```python
from build123d import *

# Parameters (mm, degrees)
F1_DEPTH = 6.35
F3_DEPTH = 3.175
F4_R     = 3.175
F5_DEPTH = 3.175


with BuildPart() as f1:
    # F0 (on Front) → F1 (new body, symmetric)
    with BuildSketch(Plane.XZ):
        with BuildLine():
            Line((0, 10.922), (0, 0))
            Line((0, 0), (10.922, 0))
            ThreePointArc((10.922, 0), (7.7230202641, 7.7230202641), (0, 10.922))
        make_face()
        with BuildLine():
            Line((10.922, 0), (0, 0))
            Line((0, 0), (0, -6.223))
            Line((0, -6.223), (8.9757648699, -6.223))
            ThreePointArc((8.9757648699, -6.223), (10.4240919966, -3.2601211704), (10.922, 0))
        make_face()
        with BuildLine():
            ThreePointArc((0, 10.922), (-7.7230202641, 7.7230202641), (-10.922, 0))
            Line((-10.922, 0), (0, 0))
            Line((0, 0), (0, 10.922))
        make_face()
        with BuildLine():
            Line((0, 0), (-10.922, 0))
            ThreePointArc((-10.922, 0), (-10.4240919966, -3.2601211704), (-8.9757648699, -6.223))
            Line((-8.9757648699, -6.223), (0, -6.223))
            Line((0, -6.223), (0, 0))
        make_face()
    extrude(amount=F1_DEPTH, both=True)

    # F2 (on face) → F3 (join)
    with BuildSketch(Plane.XZ.offset(6.35)):
        with BuildLine():
            Line((3.175, 0), (0, 0))
            Line((0, 0), (0, -3.175))
            ThreePointArc((0, -3.175), (2.2450640303, -2.2450640303), (3.175, 0))
        make_face()
        with BuildLine():
            Line((0, 3.175), (0, 0))
            Line((0, 0), (3.175, 0))
            ThreePointArc((3.175, 0), (2.2450640303, 2.2450640303), (0, 3.175))
        make_face()
        with BuildLine():
            ThreePointArc((0, 3.175), (-2.2450640303, 2.2450640303), (-3.175, 0))
            Line((-3.175, 0), (0, 0))
            Line((0, 0), (0, 3.175))
        make_face()
        with BuildLine():
            Line((0, 0), (-3.175, 0))
            ThreePointArc((-3.175, 0), (-2.2450640303, -2.2450640303), (0, -3.175))
            Line((0, -3.175), (0, 0))
        make_face()
    extrude(amount=F3_DEPTH)

    # F4 (on face) → F5 (join)
    with BuildSketch(Plane(origin=(0, 6.35, 0), x_dir=(-1, 0, 0), z_dir=(0, 1, 0))):
        Circle(F4_R)
    extrude(amount=F5_DEPTH)


solid = f1.part
```
CAD build for the part. Positions are in the model's coordinates, mm. Round coordinates to 2 decimals unless told otherwise and drop trailing zeros. Order: outer loops, then holes, each group sorted by start corner. A loop starts at its lowest first (then second) coordinate and runs counter-clockwise, first axis right, second up. Notation, with made-up numbers: (83.5, 10) - (139.5, 10) arc R29 ccw to (139.5, 32) - close; hole circle Ø5 at (84.25, 33.5). An arc over 180 degrees is marked (long way). Answer as CSV lines item,"result". Start each with the question number.
1. Saw through at A-A, the plane y = 7. Write the cut outline in (x, z) (3 decimals).
2. Pull direction Z, two halves, no side cores. Call faces 1 (the face through (0.69, 7.92, -3.1)), 2 (the face through (2.3, -6.35, 2.5)), 3 (the face through (0, 0, -6.223)): +Z half, -Z half, draft (parallel to the pull), parting line (faces both ways), or undercut.
3. Saw through at C-C, the plane x = -6.75. Write the cut outline in (y, z), and give its area (3 significant figures).
4. Saw through at D-D, the plane y = -1.75. Write the cut outline in (x, z), and give its area (3 significant figures).
5. Drill centre lines: L1, parallel to Y at x = -7, z = 4.5; L2, parallel to X at y = 2.5, z = -4.5; L3, parallel to X at y = 6.75, z = 1.75. Where is each one in solid material? Low to high. Write a range as [from, to].
6. Pin check, flat tips, straight feed: pin 1 (1.5 mm diameter, centred on x = 2, z = 7, fed in from -Y); pin 2 (1 mm diameter, centred on y = -2, z = 6, fed in from +X). Stop position of each tip, or through.
Model answer:
1,outline,"circle Ø6.35 at (0, 0)"
2,face 1,"parting line"
2,face 2,"draft"
2,face 3,"-Z half"
3,outline,"(-6.35, -6.22) - (6.35, -6.22) - (6.35, 8.59) - (-6.35, 8.59) - close"
3,area,"188 mm²"
4,outline,"(-8.98, -6.22) - (8.98, -6.22) arc R10.92 ccw (long way) to start"
4,area,"316 mm²"
5,L1,"y = [-6.35, 6.35]"
5,L2,"x = [-9.95, 9.95]"
5,L3,"x = [-2.65, 2.65]"
6,pin 1,"stops at y = -6.35"
6,pin 2,"stops at x = 9.44"
